Check sheet for the modelled part. Datum: model origin and axes. Units: mm. A direction names the side the tool comes from. Round coordinates to 2 decimals unless told otherwise and drop trailing zeros. Write each loop counter-clockwise with the first axis right and the second up, starting at its lowest first coordinate (ties: lowest second). Pieces come first, ordered by that corner, then holes. Notation, with made-up numbers: M 13,65.25 L 42,65.25 A7 ccw 42,70.25 Z; hole C 29.25,-27 d6. An arc over 180 degrees is marked long. Answer in a Markdown table with one row per item.
```python
from build123d import *

# Parameters (mm, degrees)
ESQUISSE2_R             = 4.5
ENL_V_MAT_EXTRU_1_DEPTH = 132.909059583
ESQUISSE3_W             = 90
ESQUISSE3_H             = 20
ENL_V_MAT_EXTRU_2_DEPTH = 4.5


with BuildPart() as part:
    # Esquisse1 → Base-Révolution (revolve)
    with BuildSketch(Plane.XY, mode=Mode.PRIVATE) as base_r_volution_sk:
        Polygon((0, 7), (0, 9), (1, 10), (130, 10), (130, 0), (59.041451884, 0), (55, 7), align=None)
    revolve(base_r_volution_sk.sketch.rotate(Axis((0, 0, 0), (1, 0, 0)), 90), axis=Axis((0, 0, 0), (1, 0, 0)))

    # Esquisse2 → Enlèv. mat.-Extru.1 (cut, through all)
    with BuildSketch(Plane(origin=(0, 10, 0), x_dir=(-1, 0, 0), z_dir=(0, 1, 0))):
        with Locations(Location((-120, 0, 0), (0, 0, 90))):
            Circle(ESQUISSE2_R)
    extrude(amount=-ENL_V_MAT_EXTRU_1_DEPTH, mode=Mode.SUBTRACT)

    # Esquisse3 → Enlèv. mat.-Extru.2 (cut, symmetric)
    with BuildSketch(Plane(origin=(0, 0, 0), x_dir=(1, 0, 0), z_dir=(0, 1, 0))):
        with Locations((85, 0)):
            Rectangle(ESQUISSE3_W, ESQUISSE3_H)
    extrude(amount=ENL_V_MAT_EXTRU_2_DEPTH, both=True, mode=Mode.SUBTRACT)


solid = part.part
```
1. Go/stop test with flat-tipped pins: pin 1 (5 mm diameter, centred on x = 91, y = 7.5, fed in from +Z); pin 2 (4 mm diameter, centred on x = 47.5, y = 3, fed in from +Z); pin 3 (1 mm diameter, centred on y = 3, z = 1.5, fed in from -X); pin 4 (2 mm diameter, centred on x = 62, y = 6, fed in from -Z). Record where each tip stops, or that it passes through.
Found:
| item | result |
|---|---|
| pin 1 | stops at z = 8.66 |
| pin 2 | stops at z = 8.93 |
| pin 3 | passes through |
| pin 4 | stops at z = -8.66 |
2. Section check A-A, the plane x = 120. Record the cut outline in (y, z), and give its area (3 significant figures).
Found:
| item | result |
|---|---|
| outline | M -8.93,-4.5 A10 ccw -4.5,-8.93 L -4.5,-4.5 Z; M -8.93,4.5 L -4.5,4.5 L -4.5,8.93 A10 ccw Z; M 4.5,-8.93 A10 ccw 8.93,-4.5 L 4.5,-4.5 Z; M 4.5,4.5 L 8.93,4.5 A10 ccw 4.5,8.93 Z |
| area | 47.7 mm2 |
3. Scan lines: L1, parallel to X at y = -2.5, z = -6.75; L2, parallel to Y at x = 52.5, z = -4.5; L3, parallel to Z at x = 120, y = -6.1. Record each from-to range of solid material in increasing order.
Found:
| item | result |
|---|---|
| L1 | x = 0 to 40 |
| L2 | y = -8.93 to -5.36, 5.36 to 8.93 |
| L3 | z = -7.92 to -4.5, 4.5 to 7.92 |
4. Section check C-C, the plane y = 0. Record the cut outline in (x, z), and give its area (3 significant figures).
Found:
| item | result |
|---|---|
| outline | M 0,-9 L 1,-10 L 40,-10 L 40,-7 L 0,-7 Z; M 0,7 L 40,7 L 40,10 L 1,10 L 0,9 Z |
| area | 239 mm2 |
5. Access from +Z, -Z, +X, -X, +Y, -Y to the whole of each face (thin tool, end or side, straight path). Record for faces 4 (the face through (55.87, 5.49, -0.07)), 5 (the face through (130, -7, 0)), 6 (the face through (40, 0, -8)).
Found:
| item | result |
|---|---|
| face 4 | -X |
| face 5 | +Z, -Z, +X, +Y, -Y |
| face 6 | +Z, -Z, +X |
6. Draft check along Z on faces 1 (the face through (52, 6, -8)), 2 (the face through (117.3, 7.3, -3.6)), 3 (the face through (84, 4.5, 0)). Enter one of: +Z half, -Z half, draft (parallel to the pull), parting line (faces both ways), or undercut.
Found:
| item | result |
|---|---|
| face 1 | parting line |
| face 2 | undercut |
| face 3 | draft |
7. Section check D-D, the plane x = 49.5. Record the cut outline in (y, z).
Found:
| item | result |
|---|---|
| outline | M -4.5,-8.93 L -4.5,-5.36 A7 cw -4.5,5.36 L -4.5,8.93 A10 ccw Z; M 4.5,-8.93 A10 ccw 4.5,8.93 L 4.5,5.36 A7 cw 4.5,-5.36 Z |
8. Section check B-B, the plane z = 0. Record the cut outline in (x, y).
Found:
| item | result |
|---|---|
| outline | M 0,-9 L 1,-10 L 115.5,-10 L 115.5,-4.5 L 56.44,-4.5 L 55,-7 L 0,-7 Z; M 0,7 L 55,7 L 56.44,4.5 L 115.5,4.5 L 115.5,10 L 1,10 L 0,9 Z; M 124.5,-10 L 130,-10 L 130,-4.5 L 124.5,-4.5 Z; M 124.5,4.5 L 130,4.5 L 130,10 L 124.5,10 Z |
